CAD build for the part. Positions are in the model's coordinates, mm. Coordinates: 2 decimals unless noted, no trailing zeros. Loops run counter-clockwise (first coordinate to the right, second up) from the corner with the lowest first, then second, coordinate; pieces in that order, holes last. Notation, with made-up numbers: (-17.5, 85) - (28.5, 85) arc R32 cw to (28.5, 115) - close; hole circle Ø7 at (24.25, 42). An arc over 180 degrees is marked (long way). Put each result on its own line as item: value.
```python
from build123d import *

# Parameters (mm, degrees)
F1_DEPTH = 3.175
F2_SIZE  = 3.17499


# Not quite as in the source:
# - a fillet or chamfer is up to 0.001 mm smaller than in the source, because OpenCascade refuses the exact size


with BuildPart() as f1:
    # F0 (on Front) → F1 (new body)
    with BuildSketch(Plane.XZ):
        Polygon((99.3750451773, 520.7), (0, 0), (1660.017, 0), (1560.6419548227, 520.7), align=None)
        Polygon((1535.1786987879, 13.97), (124.8383012121, 13.97), (830.0085, 205.9645134825), align=None, mode=Mode.SUBTRACT)
        Polygon((37.6746165108, 122.8850133893), (91.8845400349, 406.9312458074), (586.4115107328, 272.2879138766), align=None, mode=Mode.SUBTRACT)
        Polygon((1568.1324599651, 406.9312458074), (1622.3423834892, 122.8850133893), (1073.6054892672, 272.2879138766), align=None, mode=Mode.SUBTRACT)
        Polygon((830.0085, 338.6113142706), (212.5310268921, 506.73), (1447.4859731079, 506.73), align=None, mode=Mode.SUBTRACT)
    extrude(amount=F1_DEPTH)

    # F2 (size 3.175 in the source; OpenCascade refuses exactly that, so slightly less here)
    f2_edges = [f1.edges().sort_by_distance(p)[0] for p in [
        (64.779578, -3.175, 264.90813),
        (312.043064, -3.175, 197.586464),
        (339.148025, -3.175, 339.60958),
        (521.269763, -3.175, 422.670657),
        (830.0085, -3.175, 506.73),
        (1138.747237, -3.175, 422.670657),
        (1320.868975, -3.175, 339.60958),
        (1347.973936, -3.175, 197.586464),
        (1595.237422, -3.175, 264.90813),
        (830.0085, -3.175, 13.97),
        (1182.593599, -3.175, 109.967257),
        (477.423401, -3.175, 109.967257),
    ]]
    chamfer(f2_edges, length=F2_SIZE)


solid = f1.part
```
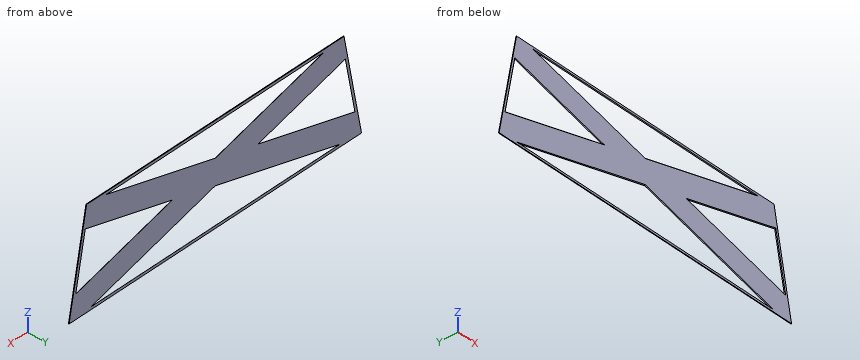
Q1. Wall check: L1, parallel to Z at x = 828, y = -2.4; L2, parallel to Z at x = 665.5, y = -1.05; L3, parallel to Z at x = 1360, y = -1.35. Give the ranges that are in metal, low to high. Write a range as from..to.
Determined:
L1: 0..11.57, 207.91..336.67, 509.13..520.7
L2: 0..12.92, 162.26..382.31, 507.78..520.7
L3: 0..12.62, 63.06..192.91, 351.66..481.51, 508.08..520.7
Q2. Slice it at B-B, the plane y = -1.4. Give the cut face in (x, z).
Determined:
outline: (0, 0) - (1660.02, 0) - (1560.64, 520.7) - (99.38, 520.7) - close; hole (35.88, 120.95) - (591.74, 272.29) - (90.79, 408.68) - close; hole (114.37, 12.57) - (1545.65, 12.57) - (830.01, 207.42) - close; hole (202.06, 508.13) - (830.01, 337.16) - (1457.96, 508.13) - close; hole (1068.28, 272.29) - (1624.14, 120.95) - (1569.22, 408.68) - close
Q3. Slice it at A-A, the plane x = 1326. State how many separate pieces and enclosed holes the cut face has, then the cut area to 3 significant figures.
Determined:
separate pieces: 4
enclosed holes: 0
area: 900 mm2
